Model file for the job. Use its own axes, mm. A direction names the side the tool comes from. Give positions to 0.01 mm unless a question says otherwise; leave off trailing zeros. Order: outer loops, then holes, each group sorted by start corner. A loop starts at its lowest first (then second) coordinate and runs counter-clockwise, first axis right, second up. Notation, with made-up numbers: (46, 53.25) - (69, 53.25) arc R13 ccw to (69, 58.25) - close; hole circle Ø6 at (55, 58). An arc over 180 degrees is marked (long way). Use CSV: the item, a comma, the result in double quotes. Start each with the question number.
(1) Probe L1, parallel to X at y = -4.25, z = -20; L2, parallel to Y at x = -20.75, z = 0; L3, parallel to Z at x = 19.5, y = 0. List the from-to ranges inside material, lowest first.
(2) Band-saw the part on A-A, the plane z = -19. Give the cut face in (x, y), then the cut area to 3 significant figures.
(3) Drop flat-ended pins along their axis: pin 1 Ø5 at (x, z) = (-20, 20) entering from -Y; pin 2 Ø3 at (x, z) = (0, 0) entering from +Y; pin 3 Ø3.5 at (x, y) = (21.5, 9) entering from -Z; pin 4 Ø3.5 at (y, z) = (12, 22) entering from -X. Give the stop position or say it passes through.
(4) Band-saw the part on B-B, the plane y = -6. Give the cut face in (x, z), then the cut area to 3 significant figures.
(5) Band-saw the part on D-D, the plane y = 1. Count the separate pieces of the cut face and the enclosed holes in it, then the cut area to 3 significant figures.
(6) Tool access for faces 4 (the flat face through (15, 11, -21)), 5 (the cylindrical face through (-16, 11, -17)), 6 (the cylindrical face through (2.11, -1.34, -19.28)): list every direction of +Z, -Z, +X, -X, +Y, -Y with a clear straight run to the whole face (end or side of a thin tool).
(7) Band-saw the part on C-C, the plane x = -19. Give the cut face in (y, z).
(8) Pull direction Y, two halves, no side cores. Call faces 1 (the conical face through (0, 7, 0)), 2 (the cylindrical face through (22, -5, -20)), 3 (the conical face through (-0.424, 0.094, -14.759)): +Y half, -Y half, draft (parallel to the pull), parting line (faces both ways), or undercut.
from build123d import *

# Parameters (mm, degrees)
SKETCH_1_W                   = 46
SKETCH_1_H                   = 46
EXTRUDE_1_DEPTH              = 15.5
CUT_EXTRUDE_1_DEPTH          = 10
SKETCH_4_R                   = 2
CUT_EXTRUDE_2_DEPTH          = 39.716921365
PATTERN_CIRCULAR_1_COUNT     = 4
HOLE_WIZARD_M6_2_D           = 5
HOLE_WIZARD_M6_2_DEPTH       = 7
HOLE_WIZARD_M6_2_CSINK_D     = 6.05
HOLE_WIZARD_M6_2_CSINK_ANGLE = 90
HOLE_WIZARD_M6_2_TIP         = 1.502151548


with BuildPart() as part:
    # 草图1 → 凸台-拉伸1 (new, symmetric)
    with BuildSketch(Plane(origin=(0, 0, 0), x_dir=(1, 0, 0), z_dir=(0, 1, 0))):
        Rectangle(SKETCH_1_W, SKETCH_1_H)
    extrude(amount=EXTRUDE_1_DEPTH, both=True)

    # 草图2 → 切除-拉伸1 (cut)
    with BuildSketch(Plane(origin=(0, 15.5, 0), x_dir=(1, 0, 0), z_dir=(0, 1, 0))):
        with BuildLine():
            Line((15, 20), (15, 23))
            Line((15, 23), (23, 23))
            Line((23, 23), (23, 15))
            Line((23, 15), (20, 15))
            ThreePointArc((20, 15), (16.464466094, 16.464466094), (15, 20))
        make_face()
        with BuildLine():
            Line((20, -15), (23, -15))
            Line((23, -15), (23, -23))
            Line((23, -23), (15, -23))
            Line((15, -23), (15, -20))
            ThreePointArc((15, -20), (16.464466094, -16.464466094), (20, -15))
        make_face()
        with BuildLine():
            Line((-15, -20), (-15, -23))
            Line((-15, -23), (-23, -23))
            Line((-23, -23), (-23, -15))
            Line((-23, -15), (-20, -15))
            ThreePointArc((-20, -15), (-16.464466094, -16.464466094), (-15, -20))
        make_face()
        with BuildLine():
            Line((-20, 15), (-23, 15))
            Line((-23, 15), (-23, 23))
            Line((-23, 23), (-15, 23))
            Line((-15, 23), (-15, 20))
            ThreePointArc((-15, 20), (-16.464466094, 16.464466094), (-20, 15))
        make_face()
    extrude(amount=-CUT_EXTRUDE_1_DEPTH, mode=Mode.SUBTRACT)

    # 草图4 → 切除-拉伸2 (cut, through all)
    with BuildSketch(Plane(origin=(0, 5.5, 0), x_dir=(1, 0, 0), z_dir=(0, 1, 0))):
        with Locations(Location((20, 20, 0), (0, 0, 270))):
            Circle(SKETCH_4_R)
        with Locations(Location((20, -20, 0), (0, 0, 270))):
            Circle(SKETCH_4_R)
        with Locations(Location((-20, -20, 0), (0, 0, 270))):
            Circle(SKETCH_4_R)
        with Locations(Location((-20, 20, 0), (0, 0, 270))):
            Circle(SKETCH_4_R)
    extrude(amount=-CUT_EXTRUDE_2_DEPTH, mode=Mode.SUBTRACT)

    # 草图6 → M6 螺纹孔1 (revolve, cut)
    with BuildSketch(Plane(origin=(0, 0, 23), x_dir=(0, -1, 0), z_dir=(1, 0, 0))):
        Polygon((0, 0), (0, 8.502151548), (2.5, 7), (2.5, 0.525), (3.025, 0), align=None)
    hole_wizard_m6_1 = revolve(axis=Axis((0, 0, 29.35), (0, 0, -1)), mode=Mode.SUBTRACT)

    # 阵列(圆周)1: M6 螺纹孔1 ×4 about axis
    pattern_circular_1_axis = Axis((0, 15.5, 0), (0, 1, 0))
    for i in range(1, PATTERN_CIRCULAR_1_COUNT):
        add(hole_wizard_m6_1.rotate(pattern_circular_1_axis, i * 360 / PATTERN_CIRCULAR_1_COUNT), mode=Mode.SUBTRACT)

    # M6 螺纹孔2
    with Locations(Plane(origin=(0, 15.5, 0), x_dir=(1, 0, 0), z_dir=(0, 1, 0))):
        with Locations((0, 0)):
            CounterSinkHole(HOLE_WIZARD_M6_2_D / 2, HOLE_WIZARD_M6_2_CSINK_D / 2, depth=HOLE_WIZARD_M6_2_DEPTH, counter_sink_angle=HOLE_WIZARD_M6_2_CSINK_ANGLE)
            with Locations((0, 0, -(HOLE_WIZARD_M6_2_DEPTH + HOLE_WIZARD_M6_2_TIP / 2))):  # 118° drill point
                Cone(0, HOLE_WIZARD_M6_2_D / 2, HOLE_WIZARD_M6_2_TIP, mode=Mode.SUBTRACT)


solid = part.part
Answer block:
1,L1,"x = -23 to -22, -18 to 18, 22 to 23"
1,L2,"y = -15.5 to -2.5, 2.5 to 15.5"
1,L3,"z = -23 to -21.94, -18.06 to -2.5, 2.5 to 18.06, 21.94 to 23"
2,outline,"(-23, -15.5) - (-21.73, -15.5) - (-21.73, 5.5) - (-23, 5.5) - close; (-18.27, -15.5) - (18.27, -15.5) - (18.27, 5.5) - (15.1, 5.5) - (15.1, 15.5) - (-15.1, 15.5) - (-15.1, 5.5) - (-18.27, 5.5) - close; (21.73, -15.5) - (23, -15.5) - (23, 5.5) - (21.73, 5.5) - close; hole circle Ø5 at (0, 0)"
2,area,"1,100 mm2"
3,pin 1,"stops at y = -15.5"
3,pin 2,"stops at y = 7.9"
3,pin 3,"stops at z = -15.01"
3,pin 4,"stops at x = -15"
4,outline,"(-23, -23) - (23, -23) - (23, 23) - (-23, 23) - close; hole circle Ø4 at (-20, -20); hole circle Ø4 at (-20, 20); hole circle Ø4 at (20, -20); hole circle Ø4 at (20, 20)"
4,area,"2,070 mm2"
5,separate pieces,"1"
5,enclosed holes,"4"
5,area,"1,930 mm2"
6,face 4,"-Z, +X, +Y"
6,face 5,"-Z, -X, +Y"
6,face 6,"-Z"
7,outline,"(-15.5, -23) - (5.5, -23) - (5.5, -21.73) - (-15.5, -21.73) - close; (-15.5, -18.27) - (5.5, -18.27) - (5.5, -15.1) - (15.5, -15.1) - (15.5, 15.1) - (5.5, 15.1) - (5.5, 18.27) - (-15.5, 18.27) - close; (-15.5, 21.73) - (5.5, 21.73) - (5.5, 23) - (-15.5, 23) - close; hole circle Ø5 at (0, 0)"
8,face 1,"+Y half"
8,face 2,"draft"
8,face 3,"undercut"
